```python
from build123d import *

# Parameters (mm, degrees)
SKETCH_1_R          = 4
EXTRUDE_1_DEPTH     = 102
SKETCH_2_W          = 10
SKETCH_2_H          = 10
EXTRUDE_2_DEPTH     = 1.5
SKETCH_6_R          = 2.055
CUT_EXTRUDE_1_DEPTH = 15
CHAMFER_1_SIZE      = 0.445
CUT_EXTRUDE_START   = 15
SKETCH_9_R          = 10
SKETCH_9_R_2        = 2.5
CUT_EXTRUDE_3_DEPTH = 88.244804269
CHAMFER1_SIZE       = 0.445


with BuildPart() as part:
    # Эскиз1 → Бобышка-Вытянуть1 (new body)
    with BuildSketch(Plane.XY):
        Circle(SKETCH_1_R)
    extrude(amount=EXTRUDE_1_DEPTH)

    # Эскиз2 → Бобышка-Вытянуть2 (add)
    with BuildSketch(Plane(origin=(0, 0, 0), x_dir=(-1, 0, 0), z_dir=(0, 0, -1))):
        Rectangle(SKETCH_2_W, SKETCH_2_H)
    extrude(amount=EXTRUDE_2_DEPTH)

    # Эскиз6 → Вырез-Вытянуть1 (cut)
    with BuildSketch(Plane(origin=(0, 0, -1.5), x_dir=(-1, 0, 0), z_dir=(0, 0, -1))):
        Circle(SKETCH_6_R)
    extrude(amount=-CUT_EXTRUDE_1_DEPTH, mode=Mode.SUBTRACT)

    # Вырез-Вытянуть2 cone 1 section (through the dimple's axis) → Вырез-Вытянуть2 (revolve, cut)
    with BuildSketch(Plane(origin=(0, 0, 13.5), x_dir=(0, 1, 0), z_dir=(1, 0, 0))):
        Polygon((0, 0), (2.055, 0), (0, 1.186454803), align=None)
    revolve(axis=Axis((0, 0, 13.5), (0, 0, 1)), mode=Mode.SUBTRACT)

    # Фаска1
    chamfer_1_edges = [part.edges().sort_by_distance(p)[0] for p in [
        (2.055, 0, -1.5),
    ]]
    chamfer(chamfer_1_edges, length=CHAMFER_1_SIZE)

    # Эскиз9 → Вырез-Вытянуть3 (cut, through all)
    with BuildSketch(Plane.XY.offset(CUT_EXTRUDE_START)):
        Circle(SKETCH_9_R)
        Circle(SKETCH_9_R_2, mode=Mode.SUBTRACT)
    extrude(amount=CUT_EXTRUDE_3_DEPTH, mode=Mode.SUBTRACT)

    # Chamfer1
    chamfer1_edges = [part.edges().sort_by_distance(p)[0] for p in [
        (-2.5, 0, 102),
    ]]
    chamfer(chamfer1_edges, length=CHAMFER1_SIZE)


solid = part.part
```
Work out the finished part from the listing and answer in its coordinate system (mm). A direction names the side the tool comes from. Give positions to 0.01 mm unless a question says otherwise; leave off trailing zeros. Write each loop counter-clockwise with the first axis right and the second up, starting at its lowest first coordinate (ties: lowest second). Pieces come first, ordered by that corner, then holes. Notation, with made-up numbers: (-34.5, -22.75) -> (-19.5, -22.75) arc R36 cw to (-19.5, 13.25) -> close; hole circle Ø3 at (48.25, 3). An arc over 180 degrees is marked (long way). Write each question's results on one line, items separated by ' | '.
1. Determine the mould class of faces 1 (the flat face through (2, 2, 15)), 2 (the cylindrical face through (0.445, -2.006, 6.121)), 3 (the cylindrical face through (-0.867, -3.905, 7.395)) for opening direction X: +X half, -X half, draft (parallel to the pull), parting line (faces both ways), or undercut.
Data:
face 1: draft | face 2: undercut | face 3: parting line
2. Find section B-B on z = 32. Determine the outline of the cut face in (x, y), and give its area (3 significant figures).
Data:
outline: circle Ø5 at (0, 0) | area: 19.6 mm^2
3. Find section A-A on z = 11.5. Determine the outline of the cut face in (x, y) (3 decimals).
Data:
outline: circle Ø8 at (0, 0); hole circle Ø4.11 at (0, 0)
4. Straight lines are drawn through the part: L1, parallel to X at y = 0, z = 5.75 (3 decimals); L2, parallel to Z at x = 2.75, y = 0.25. For each, find the intervals that lie inside material, in ascending order.
Data:
L1: -4 to -2.055, 2.055 to 4 | L2: -1.5 to 15
5. Each of these flat-tipped pins is pushed along its axis until it touches: pin 1 Ø3.5 at (x, y) = (0, 0) entering from -Z; pin 2 Ø4 at (y, z) = (-1.5, 25) entering from -X; pin 3 Ø3 at (y, z) = (-0.5, 39) entering from +X. Where does it stop, or does it pass through?
Data:
pin 1: z = 13.68 | pin 2: x = -2.5 | pin 3: x = 2.5
6. A tool of negligible diameter and unlimited length cuts with its end or side. For faces 4 (the cylindrical face through (-0.54, -2.44, 57.67)), 5 (the flat face through (0, 0, 102)), from which of +Z, -Z, +X, -X, +Y, -Y can it reach the whole face along a straight path? Write none if from no direction.
Data:
face 4: +Z | face 5: +Z, +X, -X, +Y, -Y
